```python
from build123d import *

# Parameters (mm, degrees)
BOSS_EXTRU_1_DEPTH = 1.575
BOSS_EXTRU_2_DEPTH = 1.6
BOSS_EXTRU_3_START = 10.033
BOSS_EXTRU_3_DEPTH = 10.033
BOSS_EXTRU_4_START = 1.575
BOSS_EXTRU_4_DEPTH = 1.575
BOSS_EXTRU_5_DEPTH = 9.308913653
BOSS_EXTRU_6_START = 1.6
BOSS_EXTRU_6_DEPTH = 1.6
BOSS_EXTRU_7_START = -16.383
ESQUISSE8_R        = 3.134999997
BOSS_EXTRU_7_DEPTH = 16.383


with BuildPart() as part:
    # Esquisse1 → Boss.-Extru.1 (new body)
    with BuildSketch(Plane.XZ.offset(-13.208)):
        with BuildLine():
            Line((20.6502, 3.175000004), (20.6502, 12.699999997))
            Line((20.6502, 12.699999997), (17.880200006, 11.68494557))
            Line((17.880200006, 11.68494557), (17.880200006, 2.217278617))
            ThreePointArc((17.880200006, 2.217278617), (10.55088334, -19.05), (17.880200006, -40.317278617))
            Line((17.880200006, -40.317278617), (17.880200006, -41.491086347))
            Line((17.880200006, -41.491086347), (20.6502, -41.491086347))
            Line((20.6502, -41.491086347), (20.6502, -41.275000004))
            ThreePointArc((20.6502, -41.275000004), (12.05088334, -19.05), (20.6502, 3.175000004))
        make_face()
    extrude(amount=-BOSS_EXTRU_1_DEPTH)

    # Esquisse2 → Boss.-Extru.2 (add)
    with BuildSketch(Plane(origin=(0, 14.783, 0), x_dir=(-1, 0, 0), z_dir=(0, 1, 0))):
        with BuildLine():
            Line((-14.380200006, -41.491086347), (-20.6502, -41.491086347))
            Line((-20.6502, -41.491086347), (-20.6502, -41.275000004))
            ThreePointArc((-20.6502, -41.275000004), (-12.05088334, -19.05), (-20.6502, 3.175000004))
            Line((-20.6502, 3.175000004), (-20.6502, 12.699999997))
            Line((-20.6502, 12.699999997), (-14.380200006, 10.402385822))
            Line((-14.380200006, 10.402385822), (-14.380200006, 3.391086347))
            ThreePointArc((-14.380200006, 3.391086347), (-7.05088334, -19.05), (-14.380200006, -41.491086347))
        make_face()
    extrude(amount=BOSS_EXTRU_2_DEPTH)

    # Esquisse3 → Boss.-Extru.3 (add)
    with BuildSketch(Plane.XZ.offset(-13.208).offset(BOSS_EXTRU_3_START)):
        with BuildLine():
            Line((12.971967471, -6.35), (14.59088334, -6.35))
            ThreePointArc((14.59088334, -6.35), (12.536898584, -24.69448721), (20.6502, -41.275000003))
            Line((20.6502, -41.275000003), (20.6502, -41.491086346))
            Line((20.6502, -41.491086346), (17.880200006, -41.491086346))
            Line((17.880200006, -41.491086346), (17.880200006, -40.317278616))
            ThreePointArc((17.880200006, -40.317278616), (10.90572349, -23.986826144), (12.971967471, -6.35))
        make_face()
    extrude(amount=-BOSS_EXTRU_3_DEPTH)

    # Esquisse4 → Boss.-Extru.4 (add)
    with BuildSketch(Plane.XZ.offset(-3.175).offset(BOSS_EXTRU_4_START)):
        with BuildLine():
            Line((17.880200006, -41.491086347), (17.880200006, -40.317278617))
            ThreePointArc((17.880200006, -40.317278617), (10.55088334, -19.05), (17.880200006, 2.217278617))
            Line((17.880200006, 2.217278617), (17.880200006, 11.68494557))
            Line((17.880200006, 11.68494557), (20.6502, 12.699999997))
            Line((20.6502, 12.699999997), (20.6502, 3.175000004))
            ThreePointArc((20.6502, 3.175000004), (12.05088334, -19.05), (20.6502, -41.275000004))
            Line((20.6502, -41.275000004), (20.6502, -41.491086347))
            Line((20.6502, -41.491086347), (17.880200006, -41.491086347))
        make_face()
    extrude(amount=-BOSS_EXTRU_4_DEPTH)

    # Esquisse5 → Boss.-Extru.5 (add)
    with BuildSketch(Plane(origin=(0, 0, -41.491086347), x_dir=(-1, 0, 0), z_dir=(0, 0, -1))):
        Polygon((-20.6502, 1.6), (-20.6502, 16.383), (-14.380200006, 16.383), (-14.380200006, 14.783), (-17.880200006, 14.783), (-17.880200006, 1.6), align=None)
    extrude(amount=BOSS_EXTRU_5_DEPTH)

    # Esquisse6 → Boss.-Extru.6 (add)
    with BuildSketch(Plane.XZ.offset(-1.6).offset(BOSS_EXTRU_6_START)):
        with BuildLine():
            Line((20.6502, -41.275000004), (20.6502, -50.8))
            Line((20.6502, -50.8), (14.380200006, -50.8))
            Line((14.380200006, -50.8), (14.380200006, -41.491086347))
            ThreePointArc((14.380200006, -41.491086347), (7.05088334, -19.05), (14.380200006, 3.391086347))
            Line((14.380200006, 3.391086347), (14.380200006, 10.402385822))
            Line((14.380200006, 10.402385822), (20.6502, 12.699999997))
            Line((20.6502, 12.699999997), (20.6502, 3.175000004))
            ThreePointArc((20.6502, 3.175000004), (12.05088334, -19.05), (20.6502, -41.275000004))
        make_face()
    extrude(amount=-BOSS_EXTRU_6_DEPTH)

    # Esquisse8 → Boss.-Extru.7 (add)
    with BuildSketch(Plane(origin=(0, 16.383, 0), x_dir=(1, 0, 0), z_dir=(0, 1, 0)).offset(BOSS_EXTRU_7_START)):
        with Locations((17.515200003, 50.8)):
            Circle(ESQUISSE8_R)
    extrude(amount=BOSS_EXTRU_7_DEPTH)


solid = part.part
```
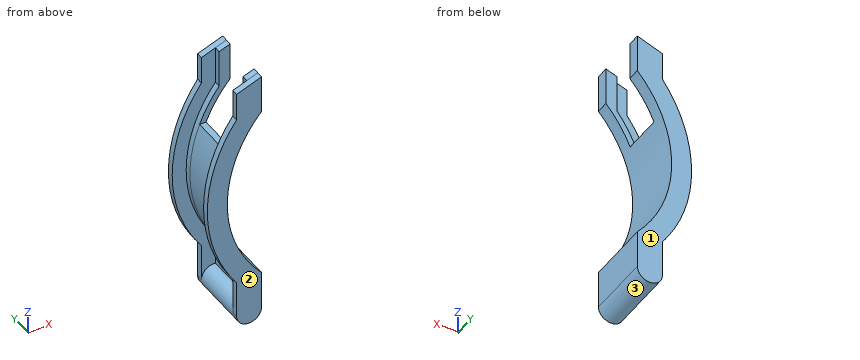
Model file for the job. Use its own axes, mm. Face numbers are marked on the shaded views. Coordinates: 2 decimals unless noted, no trailing zeros. Loops run counter-clockwise (first coordinate to the right, second up) from the corner with the lowest first, then second, coordinate; pieces in that order, holes last. Notation, with made-up numbers: M -13.5,-6.5 L 23.5,-6.5 A24 cw 23.5,27.5 Z; hole C 4,25.5 d1. An arc over 180 degrees is marked long. Use CSV: the item, a comma, the result in double quotes. Start each with the question number.
1. Flat gauge pins, fed straight in: pin 1 (1.3 mm diameter, centred on y = 1, z = 5.5, fed in from -X); pin 2 (3 mm diameter, centred on x = 12.5, y = 9.5, fed in from -Z); pin 3 (4 mm diameter, centred on x = 16.5, z = -25.5, fed in from +Y); pin 4 (0.5 mm diameter, centred on y = 2.5, z = 9, fed in from -X). Where does each tip first touch, or does it go through?
2. Band-saw the part on C-C, the plane y = 4. List the corners of the cut face in (x, z) (3 decimals), then the cut area to 3 significant figures.
3. Two-plate mould, pull along Y, no slides. Class the marked faces 1, 2 and 3: pulls with the +Y half, pulls with the -Y half, needs draft (parallel to the pull), parting line crosses it, or undercut.
4. Probe probe 1 along Y at (x, z) = (20.25, 9) (3 decimals); probe 2 along Z at (x, y) = (17, 2); probe 3 along X at (y, z) = (12.75, -19.5). List the from-to ranges inside material, lowest first. Write a range as [from, to].
5. Band-saw the part on B-B, the plane z = -14. List the corners of the cut face in (x, y) (3 decimals), then the cut area to 3 significant figures.
6. Band-saw the part on D-D, the plane z = -31.5. List the corners of the cut face in (x, y) (3 decimals).
7. Band-saw the part on A-A, the plane x = 8.5. List the corners of the cut face in (y, z).
Entries:
1,pin 1,"stops at x = 14.38"
1,pin 2,"stops at z = -34.09"
1,pin 3,"passes through"
1,pin 4,"stops at x = 17.88"
2,outline,"M 12.972,-6.35 A34.52 ccw 17.88,-40.317 L 17.88,-47.686 A3.135 ccw long 20.65,-50.8 L 20.65,-41.275 A33.02 cw 14.591,-6.35 Z"
2,area,"107 mm2"
3,face 1,"pulls with the +Y half"
3,face 2,"pulls with the -Y half"
3,face 3,"undercut"
4,probe 1,"y = [0, 3.175], [13.208, 16.383]"
4,probe 2,"z = [-53.89, -47.71], [-39.14, -36.44], [-1.66, 1.04]"
4,probe 3,"x = [10.55, 12.05]"
5,outline,"M 7.388,0 L 12.439,0 L 12.439,16.383 L 7.388,16.383 L 7.388,14.783 L 10.922,14.783 L 10.922,1.6 L 7.388,1.6 Z"
5,area,"36.2 mm2"
6,outline,"M 9.147,0 L 14.488,0 L 14.488,16.383 L 9.147,16.383 L 9.147,14.783 L 12.874,14.783 L 12.874,1.6 L 9.147,1.6 Z"
7,outline,"M 0,-29.45 L 1.6,-29.45 L 1.6,-8.65 L 0,-8.65 Z; M 14.78,-29.45 L 16.38,-29.45 L 16.38,-8.65 L 14.78,-8.65 Z"
